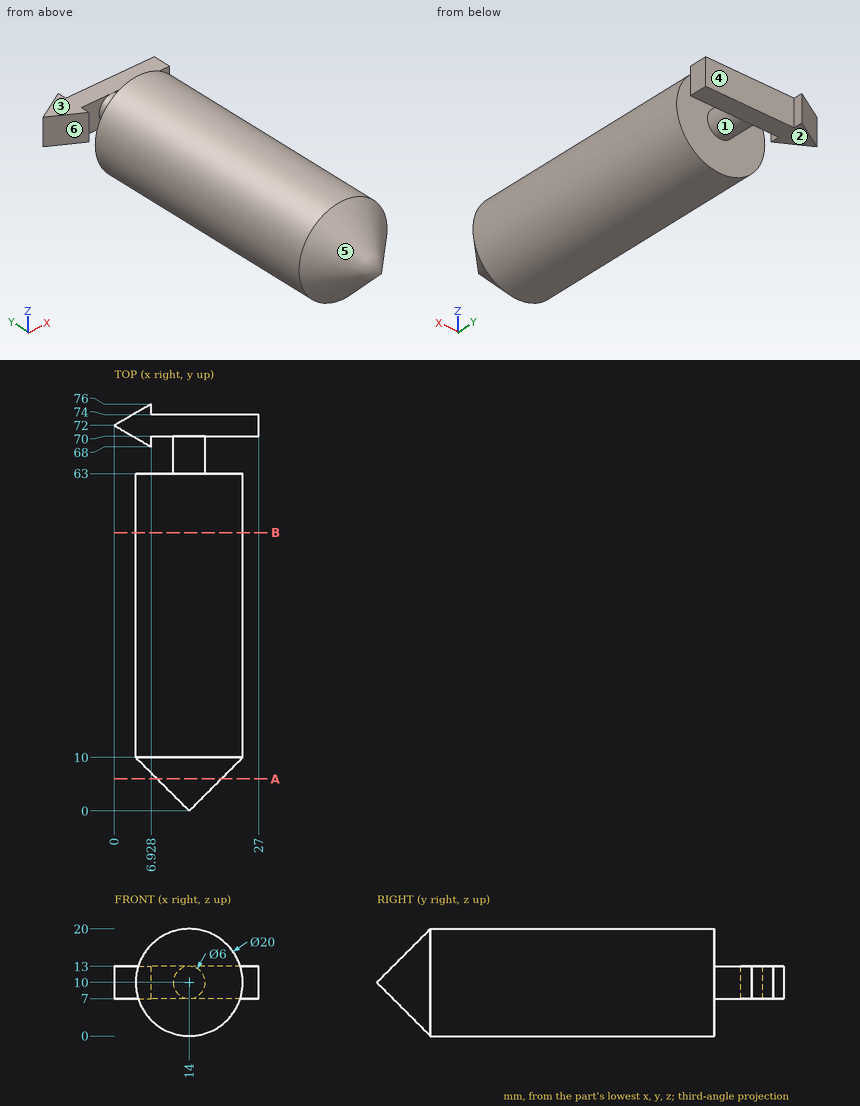
Drawing for the job (mm, zero at the part's lowest x, y, z). A direction names the side the tool comes from. Round coordinates to 2 decimals unless told otherwise and drop trailing zeros. Order: outer loops, then holes, each group sorted by start corner. A loop starts at its lowest first (then second) coordinate and runs counter-clockwise, first axis right, second up.
Item 1: Probe line 1 along X through (y, z) = (38, 10.5); line 2 along X through (y, z) = (17, 9); line 3 along Z through (x, y) = (16.75, 34.5) (1 decimal). List the from-to ranges inside material, lowest first.
Item 2: Pin check, flat tips, straight feed: pin 1 (2 mm diameter, centred on x = 5, y = 63, fed in from -Z); pin 2 (8 mm diameter, centred on x = 6, y = 10.5, fed in from +Z) (1 decimal); pin 3 (5 mm diameter, centred on x = 20, z = 10, fed in from +Y). Stop position of each tip, or through.
Item 3: Mould opens along Y. For the marked faces 4, 5 and 6 say: pulls with the +Y half, pulls with the -Y half, needs draft (parallel to the pull), parting line crosses it, or undercut.
Item 4: Saw through at A-A on y = 6. Write the cut outline in (x, z), then the cut area to 3 significant figures.
Item 5: Saw through at B-B on y = 52. Write the cut outline in (x, z).
Item 6: Tool access for the marked faces 1, 2 and 3: list every direction of +Z, -Z, +X, -X, +Y, -Y with a clear straight run to the whole face (end or side of a thin tool).
Reported:
1. line 1: x = 4.01 to 23.99
1. line 2: x = 4.05 to 23.95
1. line 3: z = 0.4 to 19.6
2. pin 1: stops at z = 4
2. pin 2: stops at z = 19.2
2. pin 3: stops at y = 74
3. face 4: pulls with the +Y half
3. face 5: pulls with the -Y half
3. face 6: undercut
4. outline: circle Ø12 at (14, 10)
4. area: 113 mm2
5. outline: circle Ø20 at (14, 10)
6. face 1: none
6. face 2: -Z, +X, -X, +Y
6. face 3: +Z, +X, -X, +Y
